```python
from build123d import *

# Parameters (mm, degrees)
SKETCH1_W           = 8
SKETCH1_H           = 28
BOSS_EXTRUDE2_DEPTH = 60
CUT_EXTRUDE2_DEPTH  = 65.353734654
SKETCH6_R           = 1.5
CUT_EXTRUDE3_DEPTH  = 25
SKETCH7_W           = 5.7
SKETCH7_H           = 3
CUT_EXTRUDE4_DEPTH  = 65.353734654
SKETCH8_R           = 1.5
CUT_EXTRUDE5_DEPTH  = 25
SKETCH9_W           = 20
SKETCH9_H           = 25
CUT_EXTRUDE6_DEPTH  = 65.353734654


with BuildPart() as part:
    # Sketch1 → Boss-Extrude2 (new body)
    with BuildSketch(Plane(origin=(0, 0, 0), x_dir=(1, 0, 0), z_dir=(0, 1, 0))):
        with Locations((6, 7.849557522)):
            Rectangle(SKETCH1_W, SKETCH1_H)
    extrude(amount=BOSS_EXTRUDE2_DEPTH)

    # Sketch5 → Cut-Extrude2 (cut, through all)
    with BuildSketch(Plane(origin=(10, 0, 0), x_dir=(0, 0, -1), z_dir=(1, 0, 0))):
        with BuildLine():
            Line((-0.087696411, 0), (15.786811455, 0))
            ThreePointArc((15.786811455, 0), (7.849557522, 7), (-0.087696411, 0))
        make_face()
    extrude(amount=-CUT_EXTRUDE2_DEPTH, mode=Mode.SUBTRACT)

    # Sketch6 → Cut-Extrude3 (cut)
    with BuildSketch(Plane.XZ):
        with Locations(Location((6, -18.349557522, 0), (0, 0, 270))):
            Circle(SKETCH6_R)
        with Locations(Location((6, 2.650442478, 0), (0, 0, 270))):
            Circle(SKETCH6_R)
    extrude(amount=-CUT_EXTRUDE3_DEPTH, mode=Mode.SUBTRACT)

    # Sketch7 → Cut-Extrude4 (cut, through all)
    with BuildSketch(Plane.ZY.offset(-2)):
        with Locations((-15.999557522, 53.5)):
            Rectangle(SKETCH7_W, SKETCH7_H)
        with Locations((0.300442478, 53.5)):
            Rectangle(SKETCH7_W, SKETCH7_H)
    extrude(amount=-CUT_EXTRUDE4_DEPTH, mode=Mode.SUBTRACT)

    # Sketch8 → Cut-Extrude5 (cut)
    with BuildSketch(Plane(origin=(0, 60, 0), x_dir=(1, 0, 0), z_dir=(0, 1, 0))):
        with Locations(Location((6, 15.999557522, 0), (0, 0, 270))):
            Circle(SKETCH8_R)
        with Locations(Location((6, -0.300442478, 0), (0, 0, 270))):
            Circle(SKETCH8_R)
    extrude(amount=-CUT_EXTRUDE5_DEPTH, mode=Mode.SUBTRACT)

    # Sketch9 → Cut-Extrude6 (cut, through all)
    with BuildSketch(Plane(origin=(10, 0, 0), x_dir=(0, 0, -1), z_dir=(1, 0, 0))):
        with Locations((3.849557522, 31.5)):
            Rectangle(SKETCH9_W, SKETCH9_H)
    extrude(amount=-CUT_EXTRUDE6_DEPTH, mode=Mode.SUBTRACT)


solid = part.part
```
Work out the finished part from the listing and answer in its coordinate system (mm). A direction names the side the tool comes from. Give positions to 0.01 mm unless a question says otherwise; leave off trailing zeros. Loops run counter-clockwise (first coordinate to the right, second up) from the corner with the lowest first, then second, coordinate; pieces in that order, holes last. Notation, with made-up numbers: (54, 27) -> (63, 27) arc R7 cw to (63, 37) -> close; hole circle Ø8 at (24, 14.25). An arc over 180 degrees is marked (long way). Write item = value, one per line. Start each with the question number.
(1) Which of the six approach directions +Z, -Z, +X, -X, +Y, -Y give full straight-line access (tool end or side, diameter ignored) to faces 1 (the flat face through (6, 53, 3.15)), 2 (the cylindrical face through (6.07, 9.37, 4.15)), 3 (the cylindrical face through (5.43, 43.62, -14.61)), 4 (the flat face through (6, 44, -4))?
(2) Find section A-A on y = 6. Give the vertices of the cut face in (x, z).
(3) Find the intervals of material crossed by probe 1 along Y at (x, z) = (4.5, 1); probe 2 along Y at (x, z) = (9, -13.75); probe 3 along Y at (x, z) = (8, 4.25), in increasing order. Write a range as from..to.
(4) Given pin 1 Ø3 at (x, z) = (8.5, -2.5) entering from -Y; pin 2 Ø2.5 at (x, z) = (6, -16) entering from +Y; pin 3 Ø2.5 at (x, z) = (6, 2.65) entering from -Y; pin 4 Ø2 at (y, z) = (20.5, -9.5) entering from -X (1 decimal), each flat-ended and moving along its own axis, determine where each tip first touches the part or whether it passes through.
(5) Find section D-D on y = 47. Give the vertices of the cut face in (x, z).
(6) The mould has two halves that part along Z. Classify faces 5 (the cylindrical face through (4.536, 48.056, -0.025)), 6 (the flat face through (2, 30, -14)), 7 (the flat face through (6, 52, 6.15)): +Z half, -Z half, draft (parallel to the pull), parting line (faces both ways), or undercut.
(7) Find section C-C on x = 3.5. Give the vertices of the cut face in (y, z), and give its area (3 significant figures).
(8) Find section B-B on z = -12.25. Give the vertices of the cut face in (x, y), and give its area (3 significant figures).
From the geometry:
q1.face_1 = +X, -X
q1.face_2 = -Y
q1.face_3 = +Y
q1.face_4 = +Z, +X, -X
q2.outline = (2, -21.85) -> (10, -21.85) -> (10, -11.72) -> (2, -11.72) -> close; (2, -3.98) -> (10, -3.98) -> (10, 6.15) -> (2, 6.15) -> close; hole circle Ø3 at (6, -18.35); hole circle Ø3 at (6, 2.65)
q3.probe_1 = 0..19, 44..52, 55..60
q3.probe_2 = 4.4..19, 44..52, 55..60
q3.probe_3 = 0..19, 44..60
q4.pin_1 = 3.13
q4.pin_2 = 35
q4.pin_3 = 44
q4.pin_4 = through
q5.outline = (2, -21.85) -> (10, -21.85) -> (10, 6.15) -> (2, 6.15) -> close; hole circle Ø3 at (6, -16); hole circle Ø3 at (6, 0.3)
q6.face_5 = undercut
q6.face_6 = draft
q6.face_7 = +Z half
q7.outline = (0, -21.85) -> (60, -21.85) -> (60, 6.15) -> (44, 6.15) -> (44, -13.85) -> (19, -13.85) -> (19, 6.15) -> (0, 6.15) -> (0, 0.09) arc R8 cw to (0, -15.79) -> close; hole (52, -18.85) -> (55, -18.85) -> (55, -13.15) -> (52, -13.15) -> close; hole (52, -2.55) -> (55, -2.55) -> (55, 3.15) -> (52, 3.15) -> close
q7.area = 1,060 mm^2
q8.outline = (2, 5.68) -> (10, 5.68) -> (10, 19) -> (2, 19) -> close; (2, 44) -> (10, 44) -> (10, 60) -> (2, 60) -> close
q8.area = 235 mm^2
